from build123d import *

# Parameters (mm, degrees)
SKETCH2_R                = 60
BOSS_EXTRUDE1_DEPTH      = 60
SKETCH3_W                = 10
SKETCH3_H                = 10.47851478
BOSS_EXTRUDE2_DEPTH      = 60
FILLET2_R                = 3
CIRPATTERN1_COUNT        = 18
FILLET2_OF_CIRPATTERN1_R = 3
SKETCH4_R                = 10
CUT_EXTRUDE1_DEPTH       = 60
SKETCH5_R                = 11.25
CUT_EXTRUDE2_DEPTH       = 60


with BuildPart() as part:
    # Sketch2 → Boss-Extrude1 (new body)
    with BuildSketch(Plane.XY):
        Circle(SKETCH2_R)
    extrude(amount=BOSS_EXTRUDE1_DEPTH)

    # Sketch3 → Boss-Extrude2 (add)
    with BuildSketch(Plane.XY.offset(60)):
        with Locations((0, 64.76074261)):
            Rectangle(SKETCH3_W, SKETCH3_H)
    boss_extrude2 = extrude(amount=-BOSS_EXTRUDE2_DEPTH)

    # Fillet2
    fillet2_edges = [part.edges().sort_by_distance(p)[0] for p in [
        (5, 70, 30),
        (0, 70, 0),
        (-5, 70, 30),
        (0, 70, 60),
    ]]
    fillet(fillet2_edges, radius=FILLET2_R)

    # CirPattern1: Boss-Extrude2 ×18 about axis
    cirpattern1_axis = Axis((0, 0, 0), (0, 0, 1))
    for i in range(1, CIRPATTERN1_COUNT):
        add(boss_extrude2.rotate(cirpattern1_axis, i * 360 / CIRPATTERN1_COUNT))

    # Fillet2 of CirPattern1
    fillet2_of_cirpattern1_edges = [part.edges().sort_by_distance(p)[0] for p in [
        (-19.242946929, 67.488584172, 30),
        (-23.941410033, 65.778483455, 0),
        (-28.639873137, 64.068382738, 30),
        (-23.941410033, 65.778483455, 60),
        (-41.164910462, 56.837049067, 30),
        (-44.995132678, 53.623111018, 0),
        (-48.825354894, 50.40917297, 30),
        (-44.995132678, 53.623111018, 60),
        (-58.121778265, 39.330127019, 30),
        (-60.621778265, 35, 0),
        (-63.121778265, 30.669872981, 30),
        (-60.621778265, 35, 60),
        (-68.068301823, 17.079411202, 30),
        (-68.936542711, 12.155372437, 0),
        (-69.804783599, 7.231333672, 30),
        (-68.936542711, 12.155372437, 60),
        (-69.804783599, -7.231333672, 30),
        (-68.936542711, -12.155372437, 0),
        (-68.068301823, -17.079411202, 30),
        (-68.936542711, -12.155372437, 60),
        (-63.121778265, -30.669872981, 30),
        (-60.621778265, -35, 0),
        (-58.121778265, -39.330127019, 30),
        (-60.621778265, -35, 60),
        (-48.825354894, -50.40917297, 30),
        (-44.995132678, -53.623111018, 0),
        (-41.164910462, -56.837049067, 30),
        (-44.995132678, -53.623111018, 60),
        (-28.639873137, -64.068382738, 30),
        (-23.941410033, -65.778483455, 0),
        (-19.242946929, -67.488584172, 30),
        (-23.941410033, -65.778483455, 60),
        (-5, -70, 30),
        (0, -70, 0),
        (5, -70, 30),
        (0, -70, 60),
        (19.242946929, -67.488584172, 30),
        (23.941410033, -65.778483455, 0),
        (28.639873137, -64.068382738, 30),
        (23.941410033, -65.778483455, 60),
        (41.164910462, -56.837049067, 30),
        (44.995132678, -53.623111018, 0),
        (48.825354894, -50.40917297, 30),
        (44.995132678, -53.623111018, 60),
        (58.121778265, -39.330127019, 30),
        (60.621778265, -35, 0),
        (63.121778265, -30.669872981, 30),
        (60.621778265, -35, 60),
        (68.068301823, -17.079411202, 30),
        (68.936542711, -12.155372437, 0),
        (69.804783599, -7.231333672, 30),
        (68.936542711, -12.155372437, 60),
        (69.804783599, 7.231333672, 30),
        (68.936542711, 12.155372437, 0),
        (68.068301823, 17.079411202, 30),
        (68.936542711, 12.155372437, 60),
        (63.121778265, 30.669872981, 30),
        (60.621778265, 35, 0),
        (58.121778265, 39.330127019, 30),
        (60.621778265, 35, 60),
        (48.825354894, 50.40917297, 30),
        (44.995132678, 53.623111018, 0),
        (41.164910462, 56.837049067, 30),
        (44.995132678, 53.623111018, 60),
        (28.639873137, 64.068382738, 30),
        (23.941410033, 65.778483455, 0),
        (19.242946929, 67.488584172, 30),
        (23.941410033, 65.778483455, 60),
    ]]
    fillet(fillet2_of_cirpattern1_edges, radius=FILLET2_OF_CIRPATTERN1_R)

    # Sketch4 → Cut-Extrude1 (cut)
    with BuildSketch(Plane.XY.offset(60)):
        Circle(SKETCH4_R)
    extrude(amount=-CUT_EXTRUDE1_DEPTH, mode=Mode.SUBTRACT)

    # Sketch5 → Cut-Extrude2 (cut)
    with BuildSketch(Plane(origin=(0, 0, 0), x_dir=(-1, 0, 0), z_dir=(0, 0, -1))):
        Circle(SKETCH5_R)
    extrude(amount=-CUT_EXTRUDE2_DEPTH, mode=Mode.SUBTRACT)


solid = part.part
Here's how the part is built. I have some questions about the finished solid (model axes, mm). A direction names the side the tool comes from. Coordinates: 2 decimals unless noted, no trailing zeros. Loops run counter-clockwise (first coordinate to the right, second up) from the corner with the lowest first, then second, coordinate; pieces in that order, holes last.
1. I need wall thicknesses on L1, parallel to Y at x = 0, z = 41.5; L2, parallel to X at y = -54.5, z = 25; L3, parallel to X at y = 50, z = 33. Which ranges of each line are inside material? Lowest first, please.
2. For faces 1 (the cylindrical face through (-10.344, 59.102, 29.58)), 2 (the cylindrical face through (-10.494, -59.075, 29.58)), 3 (the flat face through (-63.251, 6.076, 30.42)), 4 (the flat face through (63.251, 6.076, 30.42)), which set-ups out of +Z, -Z, +X, -X, +Y, -Y let a thin tool reach every point of the face, with its end or its side?
3. Imagine slicing it at C-C, the plane y = -23.5. Please give me the cut outline in (x, z), and give its area (3 significant figures).
4. Imagine slicing it at B-B, the plane x = 0. Please give me the cut outline in (y, z), and give its area (3 significant figures).
5. Imagine slicing it at A-A, the plane y = 0. Please give me the cut outline in (x, z), and give its area (3 significant figures).
6. If we mould it in two halves opening along X, with no side actions, what happens to faces 5 (the flat face through (26.36, -57.81, 30.42)), 6 (the flat face through (23.97, -65.77, 30.38)), 7 (the cylindrical face through (-44.102, 52.667, 0.524))? For each: pulls with the +X half, pulls with the -X half, needs draft (parallel to the pull), parting line crosses it, or undercut.
7. For P1, Ø5, axis at x = -42, z = 21.5, coming from the +Y side; P2, Ø6, axis at x = -27.5, z = 41, coming from the +Y side; P3, Ø12, axis at y = 54, z = 24.5, coming from the -X side, each with a flat end and sliding along its axis, tell me the tip position at first contact or that it passes through.
Taken from the geometry:
1. L1: y = -70 to -11.25, 11.25 to 70
1. L2: x = -43.95 to -39.2, -25.16 to 25.16, 39.2 to 43.95
1. L3: x = -47.6 to -35.43, -33.17 to 33.17, 35.43 to 47.6
2. face 1: +Z, -Z, +Y
2. face 2: +Z, -Z, -Y
2. face 3: +Z, -Z, -X
2. face 4: +Z, -Z, +X
3. outline: (-55.21, 0) - (55.21, 0) - (55.21, 60) - (-55.21, 60) - close
3. area: 6,620 mm2
4. outline: (-70, 3) arc R3 ccw to (-67, 0) - (-11.25, 0) - (-11.25, 60) - (-67, 60) arc R3 ccw to (-70, 57) - close; (11.25, 0) - (67, 0) arc R3 ccw to (70, 3) - (70, 57) arc R3 ccw to (67, 60) - (11.25, 60) - close
4. area: 7,040 mm2
5. outline: (-60, 0) - (-11.25, 0) - (-11.25, 60) - (-60, 60) - close; (11.25, 0) - (60, 0) - (60, 60) - (11.25, 60) - close
5. area: 5,850 mm2
6. face 5: undercut
6. face 6: pulls with the +X half
6. face 7: pulls with the -X half
7. P1: stops at y = 55.61
7. P2: stops at y = 65.58
7. P3: stops at x = -47.6
